from build123d import *

# Parameters (mm, degrees)
SKETCH_4_W           = 42
SKETCH_4_H           = 40
EXTRUDE_1_DEPTH      = 3
SKETCH_9_W           = 3
SKETCH_9_H           = 25
EXTRUDE_3_DEPTH      = 42
SKETCH_10_R          = 21
EXTRUDE_2_DEPTH      = 3
CUT_EXTRUDE_6_DEPTH  = 3
SKETCH_16_R          = 1.5
CUT_EXTRUDE_7_DEPTH  = 3
SKETCH_14_R          = 1.952306129
CUT_EXTRUDE_8_DEPTH  = 3
SKETCH_17_R          = 1.5
CUT_EXTRUDE_10_DEPTH = 3


with BuildPart() as part:
    # 草图4 → 凸台-拉伸1 (new body)
    with BuildSketch(Plane(origin=(0, 0, 0), x_dir=(1, 0, 0), z_dir=(0, 1, 0))):
        with Locations((0, -1)):
            Rectangle(SKETCH_4_W, SKETCH_4_H)
    extrude(amount=EXTRUDE_1_DEPTH)

    # 草图9 → 拉伸-薄壁3 (add)
    with BuildSketch(Plane.ZY.offset(21)):
        with Locations((-17.5, 15.5)):
            Rectangle(SKETCH_9_W, SKETCH_9_H)
    extrude(amount=-EXTRUDE_3_DEPTH)

    # 草图10 → 凸台-拉伸2 (add)
    with BuildSketch(Plane.XY.offset(-16)):
        with Locations((0, 28)):
            Circle(SKETCH_10_R)
    extrude(amount=-EXTRUDE_2_DEPTH)

    # 草图11 → 切除-拉伸6 (cut)
    with BuildSketch(Plane.XY.offset(-16)):
        with BuildLine():
            Line((-7, 37.068273953), (-7, 17.068273953))
            ThreePointArc((-7, 17.068273953), (0, 10.068273953), (7, 17.068273953))
            Line((7, 17.068273953), (7, 37.068273953))
            ThreePointArc((7, 37.068273953), (0, 44.068273953), (-7, 37.068273953))
        make_face()
    extrude(amount=-CUT_EXTRUDE_6_DEPTH, mode=Mode.SUBTRACT)

    # 草图16 → 切除-拉伸7 (cut)
    with BuildSketch(Plane.XY.offset(-16)):
        with Locations((-8.832661919, 42.279402206)):
            Circle(SKETCH_16_R)
        with Locations((-17.791157853, 26.76283209)):
            Circle(SKETCH_16_R)
        with Locations((-8.832661919, 11.246261974)):
            Circle(SKETCH_16_R)
        with Locations((9.084329947, 11.246261974)):
            Circle(SKETCH_16_R)
        with Locations((18.04282588, 26.76283209)):
            Circle(SKETCH_16_R)
        with Locations((9.084329947, 42.279402206)):
            Circle(SKETCH_16_R)
    extrude(amount=-CUT_EXTRUDE_7_DEPTH, mode=Mode.SUBTRACT)

    # 草图14 → 切除-拉伸8 (cut)
    with BuildSketch(Plane.XY.offset(-16)):
        with Locations((-8.832661919, 42.279402206)):
            Circle(SKETCH_14_R)
    extrude(amount=-CUT_EXTRUDE_8_DEPTH, mode=Mode.SUBTRACT)

    # 草图17 → 切除-拉伸10 (cut)
    with BuildSketch(Plane(origin=(0, 3, 0), x_dir=(1, 0, 0), z_dir=(0, 1, 0))):
        with Locations((-18, 13)):
            Circle(SKETCH_17_R)
        with Locations((18, 13)):
            Circle(SKETCH_17_R)
        with Locations((-18, -18)):
            Circle(SKETCH_17_R)
        with Locations((18, -18)):
            Circle(SKETCH_17_R)
    extrude(amount=-CUT_EXTRUDE_10_DEPTH, mode=Mode.SUBTRACT)


solid = part.part
Verification items for the finished model (mm, model axes). A direction names the side the tool comes from. Give positions to 0.01 mm unless a question says otherwise; leave off trailing zeros. Write each loop counter-clockwise with the first axis right and the second up, starting at its lowest first coordinate (ties: lowest second). Pieces come first, ordered by that corner, then holes. Notation, with made-up numbers: M 61.25,71.25 L 116.25,71.25 A18 cw 116.25,85.25 Z; hole C 45,-31.75 d2. An arc over 180 degrees is marked long. Use CSV: the item, a comma, the result in double quotes.
1) Cross-section at D-D (x = -18). Enter the section's corners in (y, z).
Final values:
outline,"M 0,-19 L 25.28,-19 L 25.28,-16 L 3,-16 L 3,-14.5 L 0,-14.5 Z; M 0,-11.5 L 3,-11.5 L 3,16.5 L 0,16.5 Z; M 0,19.5 L 3,19.5 L 3,21 L 0,21 Z; M 28.25,-19 L 38.82,-19 L 38.82,-16 L 28.25,-16 Z"
2) Access from +Z, -Z, +X, -X, +Y, -Y to the whole of each face (thin tool, end or side, straight path). Record for faces 5 (the face through (0, 49, -17)), 6 (the face through (0.154, 44.067, -17.479)).
Final values:
face 5,"+Z, -Z, +Y"
face 6,"+Z, -Z"
3) Release check for a two-part mould opening along Y. For faces 1 (the face through (0, 0, 1)), 2 (the face through (-7.447, 10.672, -17.479)), 3 (the face through (-21, 2.7, -6.5)), 4 (the face through (10.47, 10.67, -17.48)) record: released by +Y, released by -Y, zero draft, split by the parting line, or undercut.
Final values:
face 1,"released by -Y"
face 2,"undercut"
face 3,"zero draft"
face 4,"undercut"
4) Cross-section at C-C (x = 9). Enter the section's corners in (y, z).
Final values:
outline,"M 0,-19 L 9.75,-19 L 9.75,-16 L 3,-16 L 3,21 L 0,21 Z; M 12.74,-19 L 40.78,-19 L 40.78,-16 L 12.74,-16 Z; M 43.78,-19 L 46.97,-19 L 46.97,-16 L 43.78,-16 Z"
5) Go/stop test with flat-tipped pins: pin 1 Ø4 at (x, z) = (18, -13) entering from +Y; pin 2 Ø3 at (x, y) = (-8.83, 42.28) entering from +Z; pin 3 Ø3.5 at (x, y) = (18.04, 26.76) entering from +Z. Record where each tip stops, or that it passes through.
Final values:
pin 1,"y = 3"
pin 2,"through"
pin 3,"z = -16"
6) Cross-section at A-A (y = 19). Enter the section's corners in (x, z).
Final values:
outline,"M -21,-19 L -7,-19 L -7,-16 L -21,-16 Z; M 7,-19 L 21,-19 L 21,-16 L 7,-16 Z"
7) Cross-section at B-B (x = 0). Enter the section's corners in (y, z), plus the area to 3 significant figures.
Final values:
outline,"M 0,-19 L 10.07,-19 L 10.07,-16 L 3,-16 L 3,21 L 0,21 Z; M 44.07,-19 L 49,-19 L 49,-16 L 44.07,-16 Z"
area,"156 mm²"
8) Material ranges on line 1 along X through (y, z) = (1.2, -13); line 2 along Z through (x, y) = (10, 22); line 3 along Y through (x, z) = (4, 0.5), recorded low to high.
Final values:
line 1,"-21 to -19.5, -16.5 to 16.5, 19.5 to 21"
line 2,"-19 to -16"
line 3,"0 to 3"
